Job drawing, mm, ordinate dimensions from the low corner. One solid piece. A direction names the side the tool comes from. Round coordinates to 2 decimals unless told otherwise and drop trailing zeros. Order: outer loops, then holes, each group sorted by start corner. A loop starts at its lowest first (then second) coordinate and runs counter-clockwise, first axis right, second up. Notation, with made-up numbers: (71.25, 29) -> (95.25, 29) arc R14 cw to (95.25, 48) -> close; hole circle Ø11 at (-11.5, 49.25). An arc over 180 degrees is marked (long way). Use CSV: the item, a comma, the result in double quotes.
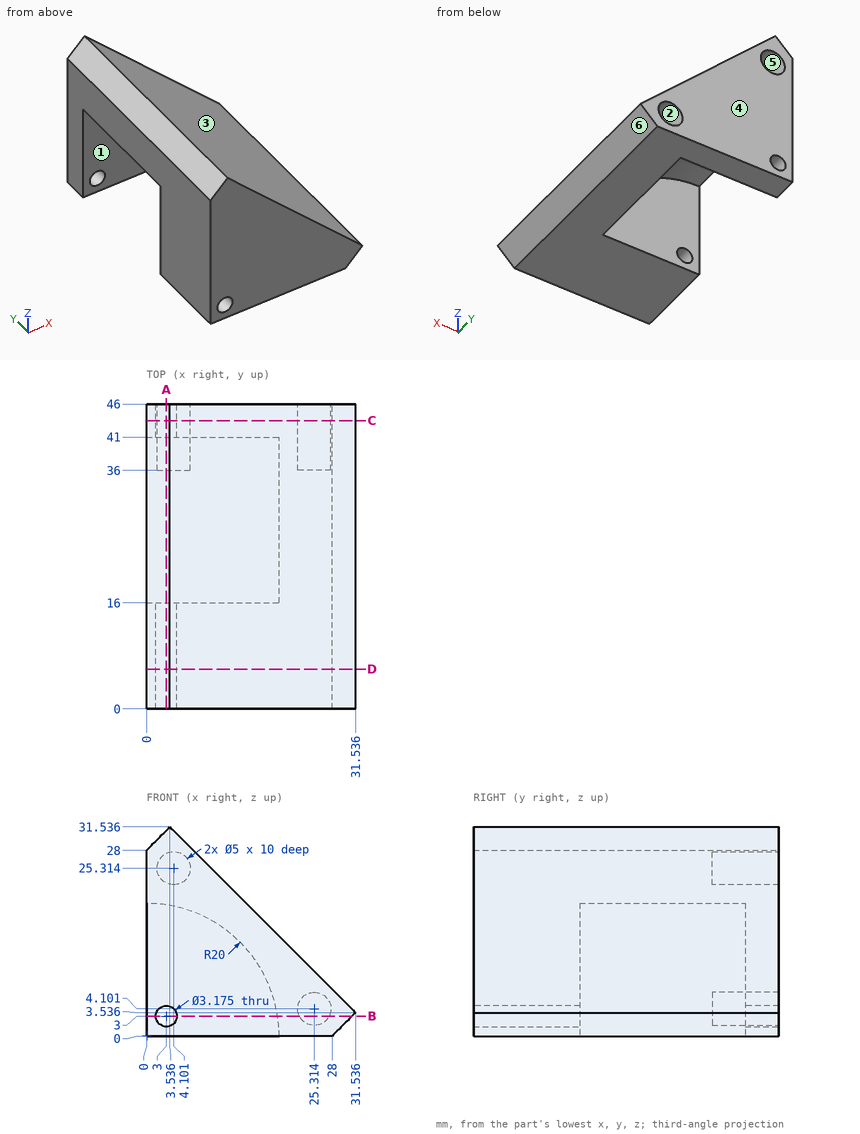
(1) Cut at A-A, the plane x = 3. Give the cut face in (y, z), then the cut area to 3 significant figures.
Reply:
outline,"(0, 0) -> (16, 0) -> (16, 1.41) -> (0, 1.41) -> close; (0, 4.59) -> (16, 4.59) -> (16, 19.77) -> (41, 19.77) -> (41, 4.59) -> (46, 4.59) -> (46, 23.07) -> (36, 23.07) -> (36, 27.56) -> (46, 27.56) -> (46, 31) -> (0, 31) -> close; (41, 0) -> (46, 0) -> (46, 1.41) -> (41, 1.41) -> close"
area,"820 mm2"
(2) Pull direction X, two halves, no side cores. Call the marked faces 4, 5 and 6: released by +X, released by -X, zero draft, split by the parting line, or undercut.
Reply:
face 4,"zero draft"
face 5,"undercut"
face 6,"released by +X"
(3) Cut at C-C, the plane y = 43.5. Give the cut face in (x, z) (1 decimal), then the cut area to 3 significant figures.
Reply:
outline,"(0, 0) -> (28, 0) -> (31.5, 3.5) -> (3.5, 31.5) -> (0, 28) -> close; hole circle Ø3.2 at (3, 3); hole circle Ø5 at (4.1, 25.3); hole circle Ø5 at (25.3, 4.1)"
area,"543 mm2"
(4) Cut at D-D, the plane y = 6. Give the cut face in (x, z) (1 decimal).
Reply:
outline,"(0, 0) -> (28, 0) -> (31.5, 3.5) -> (3.5, 31.5) -> (0, 28) -> close; hole circle Ø3.2 at (3, 3)"
(5) Drop flat-ended pins along their axis: P1, Ø6, axis at x = 22.5, y = 9, coming from the -Z side; P2, Ø1.5, axis at y = 21.5, z = 17, coming from the -X side (1 decimal); P3, Ø8, axis at y = 23.5, z = 16.5, coming from the +X side; P4, Ø2.5, axis at x = 3, z = 3, coming from the +Y side. Give the stop position or say it passes through.
Reply:
P1,"z = 0"
P2,"x = 9.2"
P3,"x = 22.57"
P4,"through"
(6) Cut at B-B, the plane z = 3. Give the cut face in (x, y), then the cut area to 3 significant figures.
Reply:
outline,"(0, 0) -> (1.41, 0) -> (1.41, 16) -> (0, 16) -> close; (0, 41) -> (1.41, 41) -> (1.41, 46) -> (0, 46) -> close; (4.59, 0) -> (31, 0) -> (31, 46) -> (27.56, 46) -> (27.56, 36) -> (23.07, 36) -> (23.07, 46) -> (4.59, 46) -> (4.59, 41) -> (19.77, 41) -> (19.77, 16) -> (4.59, 16) -> close"
area,"820 mm2"
(7) Which spindle directions (+Z, -Z, +X, -X, +Y, -Y) get a long thin tool onto all of the face, cutting with end or side? Do the marked faces 1, 2 and 3. Say none if no direction does.
Reply:
face 1,"-Z, -X"
face 2,"+Y"
face 3,"+Z, +X, +Y, -Y"
(8) Probe probe 1 along Y at (x, z) = (3, 5.5); probe 2 along X at (y, z) = (43.55, 3) (1 decimal); probe 3 along X at (y, z) = (42, 6) (1 decimal). List the from-to ranges inside material, lowest first. Write a range as [from, to].
Reply:
probe 1,"[0, 16], [41, 46]"
probe 2,"[0, 1.4], [4.6, 23.1], [27.6, 31]"
probe 3,"[0, 23.7], [26.9, 29.1]"
